```python
from build123d import *

# Parameters (mm, degrees)
F0_R      = 50
F3_DEPTH  = 50
F2_R      = 48
F4_DEPTH  = 47
F5_R      = 34.5
F6_DEPTH  = 3
F7_R      = 48
F8_DEPTH  = 1
F9_R      = 1.65
F10_DEPTH = 25
F12_SIZE  = 1.5


with BuildPart() as f3:
    # F0 (on Top) → F3 (new body)
    with BuildSketch(Plane.XY):
        Circle(F0_R)
    extrude(amount=F3_DEPTH)

    # F2 (on offset) → F4 (cut)
    with BuildSketch(Plane.XY.offset(50)):
        Circle(F2_R)
    extrude(amount=-F4_DEPTH, mode=Mode.SUBTRACT)

    # F5 (on Top) → F6 (cut)
    with BuildSketch(Plane.XY):
        Circle(F5_R)
    extrude(amount=F6_DEPTH, mode=Mode.SUBTRACT)

    # F7 (on Top) → F8 (cut)
    with BuildSketch(Plane.XY):
        Circle(F7_R)
    extrude(amount=F8_DEPTH, mode=Mode.SUBTRACT)

    # F9 (on Top) → F10 (cut)
    with BuildSketch(Plane.XY):
        with Locations((0, -41.5)):
            Circle(F9_R)
        with Locations((35.9400542571, 20.75)):
            Circle(F9_R)
        with Locations((-35.9400542571, 20.75)):
            Circle(F9_R)
    extrude(amount=F10_DEPTH, mode=Mode.SUBTRACT)

    # F12
    f12_edges = [f3.edges().sort_by_distance(p)[0] for p in [
        (-37.590054, 20.75, 1),
        (-1.65, -41.5, 1),
        (34.290054, 20.75, 1),
    ]]
    chamfer(f12_edges, length=F12_SIZE)


solid = f3.part
```
Verification items for the finished model (mm, model axes). A direction names the side the tool comes from. Coordinates: 2 decimals unless noted, no trailing zeros. Loops run counter-clockwise (first coordinate to the right, second up) from the corner with the lowest first, then second, coordinate; pieces in that order, holes last. Notation, with made-up numbers: (37, -38) -> (64, -38) arc R25 ccw to (64, -17) -> close; hole circle Ø4 at (-36.5, -12.75). An arc over 180 degrees is marked (long way). Answer in a Markdown table with one row per item.
1) Section check A-A (x = 0). Record the cut outline in (y, z).
The answers:
| item | result |
|---|---|
| outline | (-50, 0) -> (-48, 0) -> (-48, 1) -> (-44.65, 1) -> (-43.15, 2.5) -> (-43.15, 3) -> (-48, 3) -> (-48, 50) -> (-50, 50) -> close; (-39.85, 2.5) -> (-38.35, 1) -> (-34.5, 1) -> (-34.5, 3) -> (-39.85, 3) -> close; (34.5, 1) -> (48, 1) -> (48, 0) -> (50, 0) -> (50, 50) -> (48, 50) -> (48, 3) -> (34.5, 3) -> close |
2) Draft check along Y on faces 1 (the face through (-19, 45, 50)), 2 (the face through (-47.954, 2.11, 26.829)), 3 (the face through (47.69, 15.02, 24.65)). Enter one of: released by +Y, released by -Y, zero draft, split by the parting line, or undercut.
The answers:
| item | result |
|---|---|
| face 1 | zero draft |
| face 2 | undercut |
| face 3 | split by the parting line |
3) Scan lines: line 1 along Y through (x, z) = (0, 2.7); line 2 along Y through (x, z) = (0, 32); line 3 along X through (y, z) = (20, 2) (3 decimals). Record each from-to range of solid material in increasing order. Write a range as from..to.
The answers:
| item | result |
|---|---|
| line 1 | y = -50..-43.15, -39.85..-34.5, 34.5..50 |
| line 2 | y = -50..-48, 48..50 |
| line 3 | x = -45.826..-37.955, -33.925..-28.111, 28.111..33.925, 37.955..45.826 |
4) Depth check by flat-ended pin: P1, Ø3, axis at y = 38.5, z = 13.5, coming from the -X side; P2, Ø4.5, axis at x = 35.94, y = 20.75, coming from the +Z side; P3, Ø4, axis at x = 26.5, z = 40.5, coming from the +Y side. Enter the tip coordinate at first touch or a pass-through.
The answers:
| item | result |
|---|---|
| P1 | stops at x = -33.63 |
| P2 | stops at z = 3 |
| P3 | stops at y = 43.59 |
5) Section check B-B (y = 0). Record the cut outline in (x, z), and give its area (3 significant figures).
The answers:
| item | result |
|---|---|
| outline | (-50, 0) -> (-48, 0) -> (-48, 1) -> (-34.5, 1) -> (-34.5, 3) -> (-48, 3) -> (-48, 50) -> (-50, 50) -> close; (34.5, 1) -> (48, 1) -> (48, 0) -> (50, 0) -> (50, 50) -> (48, 50) -> (48, 3) -> (34.5, 3) -> close |
| area | 254 mm2 |
6) Section check C-C (z = 38). Record the cut outline in (x, y).
The answers:
| item | result |
|---|---|
| outline | circle Ø100 at (0, 0); hole circle Ø96 at (0, 0) |
7) Access from +Z, -Z, +X, -X, +Y, -Y to the whole of each face (thin tool, end or side, straight path). Record for faces 4 (the face through (14, -32, 3)), 5 (the face through (32.907, 10.363, 1.986)), 6 (the face through (0, 36, 1)).
The answers:
| item | result |
|---|---|
| face 4 | +Z |
| face 5 | +Z, -Z |
| face 6 | -Z |
8) Section check D-D (y = 20.75). Record the cut outline in (x, z).
The answers:
| item | result |
|---|---|
| outline | (-45.49, 0) -> (-43.28, 0) -> (-43.28, 1) -> (-39.09, 1) -> (-37.59, 2.5) -> (-37.59, 3) -> (-43.28, 3) -> (-43.28, 50) -> (-45.49, 50) -> close; (-34.29, 2.5) -> (-32.79, 1) -> (-27.56, 1) -> (-27.56, 3) -> (-34.29, 3) -> close; (27.56, 1) -> (32.79, 1) -> (34.29, 2.5) -> (34.29, 3) -> (27.56, 3) -> close; (37.59, 2.5) -> (39.09, 1) -> (43.28, 1) -> (43.28, 0) -> (45.49, 0) -> (45.49, 50) -> (43.28, 50) -> (43.28, 3) -> (37.59, 3) -> close |
